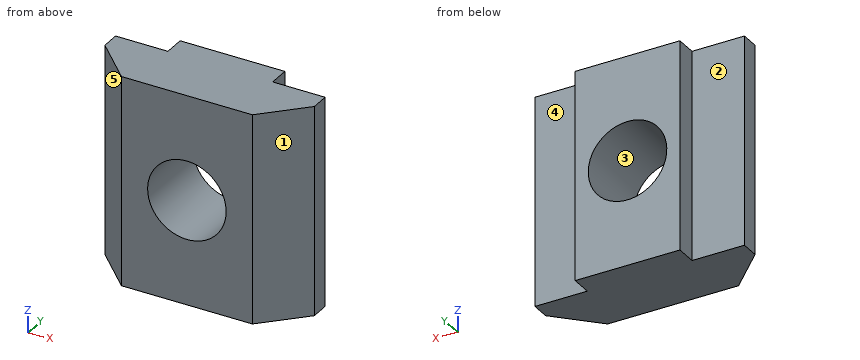
from build123d import *

# Parameters (mm, degrees)
EXTRUDE_1_DEPTH          = 16
CUT_EXTRUDE_1_DEPTH      = 19.421726303
CUT_EXTRUDE_1_DEPTH_BACK = 19.421726303
SKETCH_2_R               = 3


with BuildPart() as part:
    # 草图1 → 凸台-拉伸1 (new body)
    with BuildSketch(Plane.XY):
        Polygon((5, -4.4), (-5, -4.4), (-8, -1.4), (-8, 0), (-4, 0), (-4, 1.6), (4, 1.6), (4, 0), (8, 0), (8, -1.4), align=None)
    extrude(amount=EXTRUDE_1_DEPTH)

    # 草图2 → 切除-拉伸1 (cut, two sides: drawn at the far end of the back side and taken through both)
    with BuildSketch(Plane(origin=(0, 0, 0), x_dir=(1, 0, 0), z_dir=(0, 1, 0)).offset(-CUT_EXTRUDE_1_DEPTH_BACK)):
        with Locations(Location((0, -8, 0), (0, 0, 270))):
            Circle(SKETCH_2_R)
    extrude(amount=CUT_EXTRUDE_1_DEPTH + CUT_EXTRUDE_1_DEPTH_BACK, mode=Mode.SUBTRACT)


solid = part.part
For this review, take the finished solid that the model builds, in its own axes (mm). Face numbers are marked on the shaded views. A direction names the side the tool comes from. Round coordinates to 2 decimals unless told otherwise and drop trailing zeros. Write each loop counter-clockwise with the first axis right and the second up, starting at its lowest first coordinate (ties: lowest second). Pieces come first, ordered by that corner, then holes. Notation, with made-up numbers: M 56.5,24 L 115.5,24 A22 cw 115.5,33 Z; hole C 12,83.5 d8. An arc over 180 degrees is marked long. Write item = value, one per line. Start each with the question number.
(1) We need section D-D (z = 1.5). Give the boundary of the cut face in (x, y), then the cut area to 3 significant figures.
(2) We need section A-A (z = 8). Give the boundary of the cut face in (x, y), then the cut area to 3 significant figures.
(3) We need section C-C (y = -3.75). Give the boundary of the cut face in (x, z).
(4) Clearance check with flat-ended pins moving along their axes: pin 1 Ø2 at (x, z) = (-5.5, 6) entering from +Y; pin 2 Ø1.5 at (y, z) = (-3.5, 9) entering from -X; pin 3 Ø1 at (y, z) = (-2.5, 6) entering from +X. State where each tip first meets the part, or that it passes through.
(5) For the marked faces 1 and 2, list the 3-axis set-ups (+Z, -Z, +X, -X, +Y, -Y) from which the entire face can be reached by the end or side of a thin tool; tool diameter is ignored.
(6) We need section B-B (x = 0). Give the boundary of the cut face in (y, z).
(7) The part is to be moulded in two halves that separate along X. For the marked faces 3, 4 and 5, say which applies: +X half, -X half, draft (parallel to the pull), parting line (faces both ways), or undercut.
(8) For line 1 along Z through (x, y) = (0, -0.5); line 2 along X through (y, z) = (-0.25, 8); line 3 along X through (y, z) = (1.5, 12.5), list the stretches that pass through material, from the lowest coordinate up.
Results found:
q1.outline = M -8,-1.4 L -5,-4.4 L 5,-4.4 L 8,-1.4 L 8,0 L 4,0 L 4,1.6 L -4,1.6 L -4,0 L -8,0 Z
q1.area = 74.2 mm²
q2.outline = M -8,-1.4 L -5,-4.4 L -3,-4.4 L -3,1.6 L -4,1.6 L -4,0 L -8,0 Z; M 3,-4.4 L 5,-4.4 L 8,-1.4 L 8,0 L 4,0 L 4,1.6 L 3,1.6 Z
q2.area = 38.2 mm²
q3.outline = M -5.65,0 L 5.65,0 L 5.65,16 L -5.65,16 Z; hole C 0,8 d6
q4.pin_1 = 0
q4.pin_2 = -6.65
q4.pin_3 = 7.4
q5.face_1 = +Z, -Z, +X, -Y
q5.face_2 = +Z, -Z, -X, +Y
q6.outline = M -4.4,0 L 1.6,0 L 1.6,5 L -4.4,5 Z; M -4.4,11 L 1.6,11 L 1.6,16 L -4.4,16 Z
q7.face_3 = undercut
q7.face_4 = draft
q7.face_5 = -X half
q8.line_1 = 0 to 5, 11 to 16
q8.line_2 = -8 to -3, 3 to 8
q8.line_3 = -4 to 4
